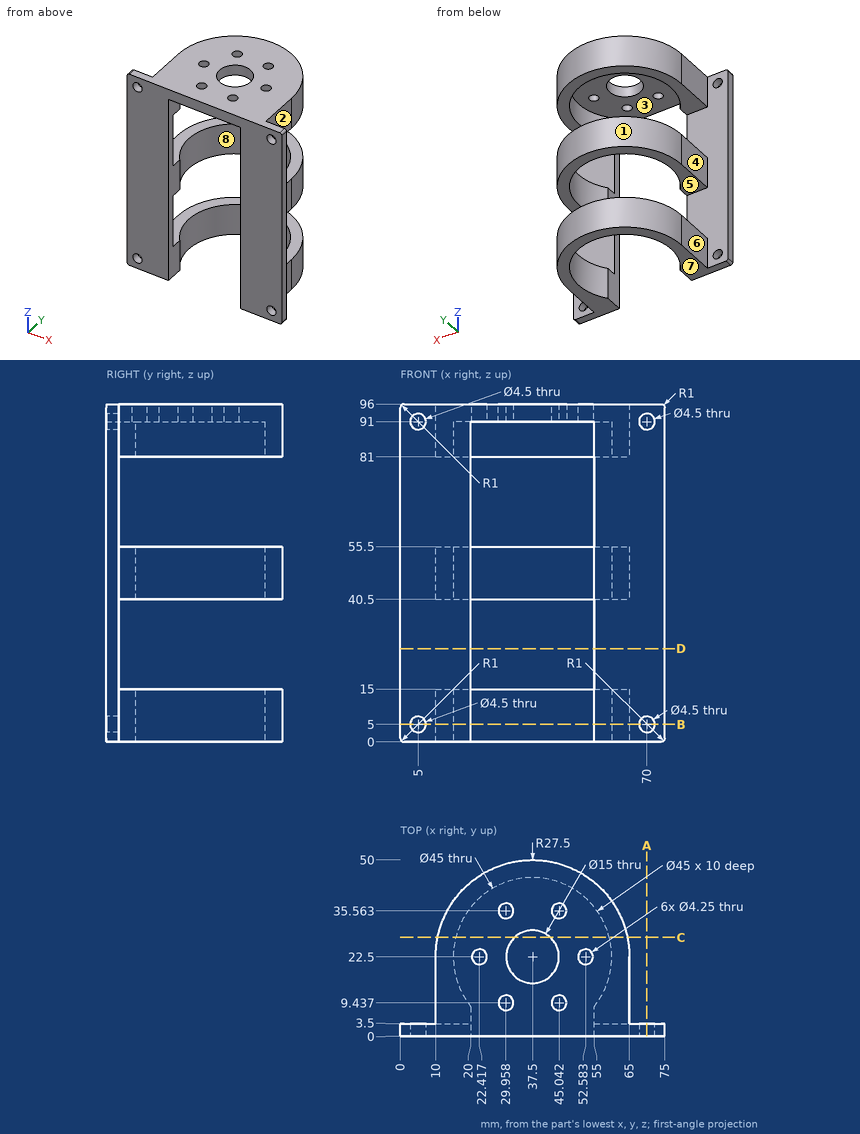
The figure shows three views and two pictorial views of one solid part (mm, origin at its lowest corner). Answer the questions. A direction names the side the tool comes from. Round coordinates to 2 decimals unless told otherwise and drop trailing zeros. Loops run counter-clockwise (first coordinate to the right, second up) from the corner with the lowest first, then second, coordinate; pieces in that order, holes last. Notation, with made-up numbers: (64.5, 43) - (97.5, 43) arc R19 ccw to (97.5, 50) - close; hole circle Ø4 at (-28, -31.5). An arc over 180 degrees is marked (long way). Use one line per item in the form item = value. Start each with the question number.
(1) Find section C-C on y = 28. Determine the outline of the cut face in (x, z) (1 decimal).
(2) Find section A-A on x = 70. Determine the outline of the cut face in (y, z).
(3) Find section D-D on z = 26.5. Determine the outline of the cut face in (x, y).
(4) Which of the six approach directions +Z, -Z, +X, -X, +Y, -Y give full straight-line access (tool end or side, diameter ignored) to the marked faces 1, 2, 3, 4 and 5?
(5) Consider line 1 (Z direction, x = 70, y = 2); line 2 (Z direction, x = 60.5, y = 21.5); line 3 (Z direction, x = 53, y = 32.5). Determine where each line is inside the solid, lowest interval first.
(6) Determine the mould class of the marked faces 6, 7 and 8 for opening direction X: +X half, -X half, draft (parallel to the pull), parting line (faces both ways), or undercut.
(7) Flat-ended cylindrical pins translate along their axes: P1, Ø6, axis at x = 39.5, y = 11.5, coming from the -Z side; P2, Ø5, axis at x = 47, z = 55, coming from the +Y side (1 decimal); P3, Ø6, axis at x = 60.5, z = 29, coming from the +Y side. Find the tip coordinate at first contact, or state that the pin passes through.
(8) Find section B-B on z = 5. Determine the outline of the cut face in (x, y).
Answer list:
q1.outline = (10.6, 0) - (15.7, 0) - (15.7, 15) - (10.6, 15) - close; (10.6, 40.5) - (15.7, 40.5) - (15.7, 55.5) - (10.6, 55.5) - close; (10.6, 81) - (15.7, 81) - (15.7, 91) - (32.4, 91) - (32.4, 96) - (10.6, 96) - close; (42.6, 91) - (59.3, 91) - (59.3, 81) - (64.4, 81) - (64.4, 96) - (42.6, 96) - close; (59.3, 0) - (64.4, 0) - (64.4, 15) - (59.3, 15) - close; (59.3, 40.5) - (64.4, 40.5) - (64.4, 55.5) - (59.3, 55.5) - close
q2.outline = (0, 0) - (3.5, 0) - (3.5, 2.75) - (0, 2.75) - close; (0, 7.25) - (3.5, 7.25) - (3.5, 88.75) - (0, 88.75) - close; (0, 93.25) - (3.5, 93.25) - (3.5, 96) - (0, 96) - close
q3.outline = (0, 0) - (20, 0) - (20, 3.5) - (0, 3.5) - close; (55, 0) - (75, 0) - (75, 3.5) - (55, 3.5) - close
q4.face_1 = +Z, -Z, +Y
q4.face_2 = +Z, -Z, +X, +Y
q4.face_3 = -Z
q4.face_4 = +Z, -Z, -X, +Y
q4.face_5 = +X, -X, +Y
q5.line_1 = 0 to 2.75, 7.25 to 88.75, 93.25 to 96
q5.line_2 = 0 to 15, 40.5 to 55.5, 81 to 96
q5.line_3 = 91 to 96
q6.face_6 = -X half
q6.face_7 = draft
q6.face_8 = undercut
q7.P1 = 91
q7.P2 = 49.1
q7.P3 = 3.5
q8.outline = (0, 0) - (2.75, 0) - (2.75, 3.5) - (0, 3.5) - close; (7.25, 0) - (20, 0) - (20, 8.36) arc R22.5 cw (long way) to (55, 8.36) - (55, 0) - (67.75, 0) - (67.75, 3.5) - (65, 3.5) - (65, 22.5) arc R27.5 ccw to (10, 22.5) - (10, 3.5) - (7.25, 3.5) - close; (72.25, 0) - (75, 0) - (75, 3.5) - (72.25, 3.5) - close
